```python
from build123d import *

# Parameters (mm, degrees)
SKETCH1_R           = 30
BOSS_EXTRUDE1_DEPTH = 15
SKETCH3_R           = 16.25
CUT_EXTRUDE1_DEPTH  = 5
SKETCH4_R           = 7
CUT_EXTRUDE2_DEPTH  = 11
SKETCH5_R           = 30
SKETCH5_R_2         = 17.5
CUT_EXTRUDE3_DEPTH  = 5
SKETCH6_R           = 2
CUT_EXTRUDE4_DEPTH  = 11


with BuildPart() as part:
    # Sketch1 → Boss-Extrude1 (new body)
    with BuildSketch(Plane(origin=(0, 0, 0), x_dir=(1, 0, 0), z_dir=(0, 1, 0))):
        Circle(SKETCH1_R)
    extrude(amount=BOSS_EXTRUDE1_DEPTH)

    # Sketch3 → Cut-Extrude1 (cut)
    with BuildSketch(Plane.XZ):
        Circle(SKETCH3_R)
    extrude(amount=-CUT_EXTRUDE1_DEPTH, mode=Mode.SUBTRACT)

    # Sketch4 → Cut-Extrude2 (cut, through all)
    with BuildSketch(Plane.XZ.offset(-5)):
        Circle(SKETCH4_R)
    extrude(amount=-CUT_EXTRUDE2_DEPTH, mode=Mode.SUBTRACT)

    # Sketch5 → Cut-Extrude3 (cut)
    with BuildSketch(Plane(origin=(0, 15, 0), x_dir=(1, 0, 0), z_dir=(0, 1, 0))):
        Circle(SKETCH5_R)
        Circle(SKETCH5_R_2, mode=Mode.SUBTRACT)
    extrude(amount=-CUT_EXTRUDE3_DEPTH, mode=Mode.SUBTRACT)

    # Sketch6 → Cut-Extrude4 (cut, through all)
    with BuildSketch(Plane(origin=(0, 10, 0), x_dir=(1, 0, 0), z_dir=(0, 1, 0))):
        with Locations((0, 23.5)):
            Circle(SKETCH6_R)
        with Locations((20.351596989, 11.75)):
            Circle(SKETCH6_R)
        with Locations((20.351596989, -11.75)):
            Circle(SKETCH6_R)
        with Locations((0, -23.5)):
            Circle(SKETCH6_R)
        with Locations((-20.351596989, -11.75)):
            Circle(SKETCH6_R)
        with Locations((-20.351596989, 11.75)):
            Circle(SKETCH6_R)
    extrude(amount=-CUT_EXTRUDE4_DEPTH, mode=Mode.SUBTRACT)


solid = part.part
```
Work out the finished part from the listing and answer in its coordinate system (mm). A direction names the side the tool comes from. Give positions to 0.01 mm unless a question says otherwise; leave off trailing zeros. Loops run counter-clockwise (first coordinate to the right, second up) from the corner with the lowest first, then second, coordinate; pieces in that order, holes last. Notation, with made-up numbers: M 52,-13.5 L 60,-13.5 A25 cw 60,15.5 Z; hole C -19.5,12.5 d9. An arc over 180 degrees is marked long. One line per item, written item: value. Start each with the question number.
1. Find section C-C (z = -11.75). Give the vertices of the cut face in (x, y).
2. Find section A-A (y = 6.75). Give the vertices of the cut face in (x, z).
3. Find section D-D (x = -20). Give the vertices of the cut face in (y, z).
4. Find the intervals of material crossed by probe 1 along Z at (x, y) = (0, 4.5); probe 2 along Z at (x, y) = (0, 9.5); probe 3 along X at (y, z) = (6.25, 11.75), in increasing order.
5. Find section B-B (x = 6). Give the vertices of the cut face in (y, z), and give its area (3 significant figures).
6. Which of the six approach directions +Z, -Z, +X, -X, +Y, -Y give full straight-line access (tool end or side, diameter ignored) to faces 5 (the face through (15.5, 2.46, 4.88)), 6 (the face through (0, 15, 8)), 7 (the face through (13, 10, 13))?
7. Each of these flat-tipped pins is pushed along its axis until it touches: P1, Ø2, axis at y = 8, z = -6, coming from the -X side; P2, Ø3.5, axis at x = -20.35, z = 11.75, coming from the +Y side; P3, Ø1.5, axis at y = 9, z = 18.5, coming from the -X side; P4, Ø6, axis at y = 5.5, z = -5.5, coming from the +X side. Where does it stop, or does it pass through?
8. Determine the mould class of faces 1 (the face through (-13.887, 12.535, 10.648)), 2 (the face through (7, 5, -3)), 3 (the face through (13, 0, 13)), 4 (the face through (-18.444, 5.07, -12.351)) for opening direction X: released by +X, released by -X, zero draft, split by the parting line, or undercut.
Reported:
1. outline: M -27.6,0 L -22.35,0 L -22.35,10 L -27.6,10 Z; M -18.35,0 L -11.22,0 L -11.22,5 L 11.22,5 L 11.22,0 L 18.35,0 L 18.35,10 L 12.97,10 L 12.97,15 L -12.97,15 L -12.97,10 L -18.35,10 Z; M 22.35,0 L 27.6,0 L 27.6,10 L 22.35,10 Z
2. outline: C 0,0 d60; hole C -20.35,-11.75 d4; hole C -20.35,11.75 d4; hole C 0,0 d14; hole C 0,-23.5 d4; hole C 0,23.5 d4; hole C 20.35,-11.75 d4; hole C 20.35,11.75 d4
3. outline: M 0,-22.36 L 10,-22.36 L 10,-13.72 L 0,-13.72 Z; M 0,-9.78 L 10,-9.78 L 10,9.78 L 0,9.78 Z; M 0,13.72 L 10,13.72 L 10,22.36 L 0,22.36 Z
4. probe 1: z = -30 to -25.5, -21.5 to -16.25, 16.25 to 21.5, 25.5 to 30
4. probe 2: z = -30 to -25.5, -21.5 to -7, 7 to 21.5, 25.5 to 30
4. probe 3: x = -27.6 to -22.35, -18.35 to 18.35, 22.35 to 27.6
5. outline: M 0,-29.39 L 10,-29.39 L 10,-16.44 L 15,-16.44 L 15,-3.61 L 5,-3.61 L 5,-15.1 L 0,-15.1 Z; M 0,15.1 L 5,15.1 L 5,3.61 L 15,3.61 L 15,16.44 L 10,16.44 L 10,29.39 L 0,29.39 Z
5. area: 529 mm²
6. face 5: -Y
6. face 6: +Z, -Z, +X, -X, +Y
6. face 7: +Y
7. P1: stops at x = -29.58
7. P2: passes through
7. P3: stops at x = -24.19
7. P4: stops at x = 29.9
8. face 1: split by the parting line
8. face 2: undercut
8. face 3: zero draft
8. face 4: undercut
